Input: part model. Units: mm. Frame: model coordinates. A direction names the side the tool comes from. Round coordinates to 2 decimals unless told otherwise and drop trailing zeros. Loops run counter-clockwise (first coordinate to the right, second up) from the corner with the lowest first, then second, coordinate; pieces in that order, holes last.
(1) Line query: line 1 (Z direction, x = -12.7, y = -1.3); line 2 (X direction, y = -2.15, z = 57.15); line 3 (Y direction, x = -74.2, z = 38.1) (3 decimals). Output: solid intervals per line, ascending.
(2) Cut plane B-B, the plane z = 25.4. Output: boundary loops of the cut face in (x, y) (3 decimals), and give its area (3 significant figures).
(3) Draft query along Z for faces 3 (the face through (-12.326, -1.61, 58.836)), 4 (the face through (-75, -25.4, 38)), 5 (the face through (-47, -2, 0)), 6 (the face through (-47, -2, 76.2)). Return one class per face: released by +Z, released by -Z, zero draft, split by the parting line, or undercut.
(4) Cut plane D-D, the plane y = -5. Output: boundary loops of the cut face in (x, z) (3 decimals), and give its area (3 significant figures).
(5) Cut plane A-A, the plane x = -12.7. Output: boundary loops of the cut face in (y, z) (3 decimals).
(6) Access query for faces 1 (the face through (-12.475, -1.61, 36.387)), 2 (the face through (-73.025, -10, 38)). Directions: +Z, -Z, +X, -X, +Y, -Y. A direction counts if a zero-diameter tool reaches every point of the face in a straight line with its end or side. Return the directions, or none.
(7) Cut plane C-C, the plane z = 38.1. Output: boundary loops of the cut face in (x, y) (3 decimals), and give its area (3 significant figures).
(8) First-contact query: pin 1 Ø10 at (y, z) = (-15.24, 38.1) entering from +X (3 decimals); pin 2 Ø6 at (x, z) = (-61.5, 28) entering from -Y (3 decimals). Flat tips, straight axial feed; report the tip coordinate or a pass-through.
from build123d import *

# Parameters (mm, degrees)
BOSS_EXTRUDE1_DEPTH       = 76.2
CUT_EXTRUDE1_REACH        = 112.716
SKETCH8_R                 = 3.175
TAP_DRILL_FOR_8_32_TAP1_D = 3.4544
TAP_DRILL_FOR_8_32_TAP2_D = 3.4544


with BuildPart() as part:
    # Sketch2 → Boss-Extrude1 (new body)
    with BuildSketch(Plane.XY):
        Polygon((0, 0), (-76.2, 0), (-76.2, -25.4), (-73.025, -25.4), (-73.025, -3.175), (0, -3.175), align=None)
    extrude(amount=BOSS_EXTRUDE1_DEPTH)

    # Sketch8 → Cut-Extrude1 (cut, up to next)
    with BuildSketch(Plane.ZY.offset(76.2), mode=Mode.PRIVATE) as cut_extrude1_sk1:
        with Locations((38.1, -15.24)):
            Circle(SKETCH8_R)
    cut_extrude1_tool1 = extrude(cut_extrude1_sk1.sketch, amount=-CUT_EXTRUDE1_REACH, mode=Mode.PRIVATE) & part.part
    add(cut_extrude1_tool1.solids().sort_by_distance((-76.2, -15.24, 38.1))[0], mode=Mode.SUBTRACT)

    # Tap Drill for #8-32 Tap1 (through all)
    with Locations(Plane(origin=(0, 0, 0), x_dir=(1, 0, 0), z_dir=(0, 1, 0))):
        with Locations((-12.7, -38.1), (-12.7, -19.05), (-12.7, -57.15)):
            Hole(TAP_DRILL_FOR_8_32_TAP1_D / 2)

    # Tap Drill for #8-32 Tap2 (through all)
    with Locations(Plane.ZY.offset(76.2)):
        with Locations((25.4, -15.24), (50.8, -15.24)):
            Hole(TAP_DRILL_FOR_8_32_TAP2_D / 2)


solid = part.part
Reported:
1. line 1: z = 0 to 17.32, 20.78 to 36.37, 39.83 to 55.42, 58.88 to 76.2
1. line 2: x = -76.2 to -14.43, -10.97 to 0
1. line 3: y = -25.4 to -18.415, -12.065 to 0
2. outline: (-76.2, -25.4) - (-73.025, -25.4) - (-73.025, -16.967) - (-76.2, -16.967) - close; (-76.2, -13.513) - (-73.025, -13.513) - (-73.025, -3.175) - (0, -3.175) - (0, 0) - (-76.2, 0) - close
2. area: 302 mm2
3. face 3: undercut
3. face 4: zero draft
3. face 5: released by -Z
3. face 6: released by +Z
4. outline: (-76.2, 0) - (-73.025, 0) - (-73.025, 76.2) - (-76.2, 76.2) - close
4. area: 242 mm2
5. outline: (-3.175, 0) - (0, 0) - (0, 17.323) - (-3.175, 17.323) - close; (-3.175, 20.777) - (0, 20.777) - (0, 36.373) - (-3.175, 36.373) - close; (-3.175, 39.827) - (0, 39.827) - (0, 55.423) - (-3.175, 55.423) - close; (-3.175, 58.877) - (0, 58.877) - (0, 76.2) - (-3.175, 76.2) - close
6. face 1: +Y, -Y
6. face 2: +Z, -Z, +X, -Y
7. outline: (-76.2, -25.4) - (-73.025, -25.4) - (-73.025, -18.415) - (-76.2, -18.415) - close; (-76.2, -12.065) - (-73.025, -12.065) - (-73.025, -3.175) - (-14.427, -3.175) - (-14.427, 0) - (-76.2, 0) - close; (-10.973, -3.175) - (0, -3.175) - (0, 0) - (-10.973, 0) - close
7. area: 281 mm2
8. pin 1: stops at x = -73.025
8. pin 2: stops at y = -3.175
